Read the model definition and answer for the solid it produces. Units are mm, in the model's axes. Coordinates: 2 decimals unless noted, no trailing zeros. Loops run counter-clockwise (first coordinate to the right, second up) from the corner with the lowest first, then second, coordinate; pieces in that order, holes last. Notation, with made-up numbers: M -36.75,-23 L -0.75,-23 A16 ccw -0.75,-11 Z; hole C -13,24 d10. An arc over 180 degrees is marked long. One line per item, written item: value. Start each with the question number.
1. Flat-ended cylindrical pins translate along their axes: pin 1 (3 mm diameter, centred on x = 7, z = 5.5, fed in from -Y); pin 2 (12 mm diameter, centred on x = -2.5, y = -2.5, fed in from +Z); pin 3 (1.5 mm diameter, centred on y = -8, z = 1.5, fed in from -X). Find the tip coordinate at first contact, or state that the pin passes through.
2. The part is cut by section D-D (y = -3). State how many separate pieces and enclosed holes the cut face has, then the cut area to 3 significant figures.
3. Determine the mould class of faces 1 (the face through (-7, -11, 10)), 2 (the face through (-2.764, -12.447, 4.93)) for opening direction Y: +Y half, -Y half, draft (parallel to the pull), parting line (faces both ways), or undercut.
4. The part is cut by section A-A (x = 0). Write down the section's boundary in (y, z).
5. The part is cut by section C-C (x = 8.25). Write down the section's boundary in (y, z).
6. Consider probe 1 along Y at (x, z) = (0, 2.5); probe 2 along X at (y, z) = (4.5, 8); probe 3 along Z at (x, y) = (8, 7.75). Determine where each line is inside the solid, lowest interval first.
```python
from build123d import *

# Parameters (mm, degrees)
SKETCH1_R           = 15
SKETCH1_R_2         = 12.75
BOSS_EXTRUDE1_DEPTH = 10
SKETCH2_R           = 15
BOSS_EXTRUDE2_DEPTH = 0.25
FILLET1_R           = 3


with BuildPart() as part:
    # Sketch1 → Boss-Extrude1 (new body)
    with BuildSketch(Plane.XY):
        Circle(SKETCH1_R)
        Circle(SKETCH1_R_2, mode=Mode.SUBTRACT)
    extrude(amount=BOSS_EXTRUDE1_DEPTH)

    # Sketch2 → Boss-Extrude2 (add)
    with BuildSketch(Plane.XY):
        Circle(SKETCH2_R)
        with BuildLine():
            Line((5.922042758, 5.03811235), (5.03811235, 5.922042758))
            Line((5.03811235, 5.922042758), (1.502578444, 9.457576664))
            ThreePointArc((1.502578444, 9.457576664), (1.149025054, 9.457576664), (1.149025054, 9.104023274))
            Line((1.149025054, 9.104023274), (4.684558959, 5.568489368))
            Line((4.684558959, 5.568489368), (5.568489368, 4.684558959))
            Line((5.568489368, 4.684558959), (9.104023274, 1.149025054))
            ThreePointArc((9.104023274, 1.149025054), (9.457576664, 1.149025054), (9.457576664, 1.502578444))
            Line((9.457576664, 1.502578444), (5.922042758, 5.03811235))
        make_face(mode=Mode.SUBTRACT)
        with BuildLine():
            Line((6.346306827, 5.462376419), (9.881840733, 1.926842513))
            ThreePointArc((9.881840733, 1.926842513), (9.881840733, 0.724760985), (8.679759205, 0.724760985))
            Line((8.679759205, 0.724760985), (5.144225299, 4.260294891))
            Line((5.144225299, 4.260294891), (4.684605891, 3.800675483))
            ThreePointArc((4.684605891, 3.800675483), (6.032467694, 0), (4.684605891, -3.800675483))
            Line((4.684605891, -3.800675483), (5.144225299, -4.260294891))
            Line((5.144225299, -4.260294891), (8.679759205, -0.724760985))
            ThreePointArc((8.679759205, -0.724760985), (9.881840733, -0.724760985), (9.881840733, -1.926842513))
            Line((9.881840733, -1.926842513), (6.346306827, -5.462376419))
            Line((6.346306827, -5.462376419), (6.805926235, -5.921995827))
            Line((6.805926235, -5.921995827), (12.727922061, 0))
            Line((12.727922061, 0), (6.805926235, 5.921995827))
            Line((6.805926235, 5.921995827), (6.346306827, 5.462376419))
        make_face(mode=Mode.SUBTRACT)
        with BuildLine():
            Line((5.462376419, 6.346306827), (1.926842513, 9.881840733))
            ThreePointArc((1.926842513, 9.881840733), (0.724760985, 9.881840733), (0.724760985, 8.679759205))
            Line((0.724760985, 8.679759205), (4.260294891, 5.144225299))
            Line((4.260294891, 5.144225299), (3.800675483, 4.684605891))
            ThreePointArc((3.800675483, 4.684605891), (0, 6.032467694), (-3.800675483, 4.684605891))
            Line((-3.800675483, 4.684605891), (-4.260294891, 5.144225299))
            Line((-4.260294891, 5.144225299), (-0.724760985, 8.679759205))
            ThreePointArc((-0.724760985, 8.679759205), (-0.724760985, 9.881840733), (-1.926842513, 9.881840733))
            Line((-1.926842513, 9.881840733), (-5.462376419, 6.346306827))
            Line((-5.462376419, 6.346306827), (-5.921995827, 6.805926235))
            Line((-5.921995827, 6.805926235), (0, 12.727922061))
            Line((0, 12.727922061), (5.921995827, 6.805926235))
            Line((5.921995827, 6.805926235), (5.462376419, 6.346306827))
        make_face(mode=Mode.SUBTRACT)
        with BuildLine():
            Line((-5.568489368, 4.684558959), (-9.104023274, 1.149025054))
            ThreePointArc((-9.104023274, 1.149025054), (-9.457576664, 1.149025054), (-9.457576664, 1.502578444))
            Line((-9.457576664, 1.502578444), (-5.922042758, 5.03811235))
            Line((-5.922042758, 5.03811235), (-5.03811235, 5.922042758))
            Line((-5.03811235, 5.922042758), (-1.502578444, 9.457576664))
            ThreePointArc((-1.502578444, 9.457576664), (-1.149025054, 9.457576664), (-1.149025054, 9.104023274))
            Line((-1.149025054, 9.104023274), (-4.684558959, 5.568489368))
            Line((-4.684558959, 5.568489368), (-5.568489368, 4.684558959))
        make_face(mode=Mode.SUBTRACT)
        with BuildLine():
            Line((-6.346306827, 5.462376419), (-6.805926235, 5.921995827))
            Line((-6.805926235, 5.921995827), (-12.727922061, 0))
            Line((-12.727922061, 0), (-6.805926235, -5.921995827))
            Line((-6.805926235, -5.921995827), (-6.346306827, -5.462376419))
            Line((-6.346306827, -5.462376419), (-9.881840733, -1.926842513))
            ThreePointArc((-9.881840733, -1.926842513), (-9.881840733, -0.724760985), (-8.679759205, -0.724760985))
            Line((-8.679759205, -0.724760985), (-5.144225299, -4.260294891))
            Line((-5.144225299, -4.260294891), (-4.684605891, -3.800675483))
            ThreePointArc((-4.684605891, -3.800675483), (-6.032467694, 0), (-4.684605891, 3.800675483))
            Line((-4.684605891, 3.800675483), (-5.144225299, 4.260294891))
            Line((-5.144225299, 4.260294891), (-8.679759205, 0.724760985))
            ThreePointArc((-8.679759205, 0.724760985), (-9.881840733, 0.724760985), (-9.881840733, 1.926842513))
            Line((-9.881840733, 1.926842513), (-6.346306827, 5.462376419))
        make_face(mode=Mode.SUBTRACT)
        with BuildLine():
            Line((5.462376419, -6.346306827), (5.921995827, -6.805926235))
            Line((5.921995827, -6.805926235), (0, -12.727922061))
            Line((0, -12.727922061), (-5.921995827, -6.805926235))
            Line((-5.921995827, -6.805926235), (-5.462376419, -6.346306827))
            Line((-5.462376419, -6.346306827), (-1.926842513, -9.881840733))
            ThreePointArc((-1.926842513, -9.881840733), (-0.724760985, -9.881840733), (-0.724760985, -8.679759205))
            Line((-0.724760985, -8.679759205), (-4.260294891, -5.144225299))
            Line((-4.260294891, -5.144225299), (-3.800675483, -4.684605891))
            ThreePointArc((-3.800675483, -4.684605891), (0, -6.032467694), (3.800675483, -4.684605891))
            Line((3.800675483, -4.684605891), (4.260294891, -5.144225299))
            Line((4.260294891, -5.144225299), (0.724760985, -8.679759205))
            ThreePointArc((0.724760985, -8.679759205), (0.724760985, -9.881840733), (1.926842513, -9.881840733))
            Line((1.926842513, -9.881840733), (5.462376419, -6.346306827))
        make_face(mode=Mode.SUBTRACT)
        with BuildLine():
            Line((5.568489368, -4.684558959), (9.104023274, -1.149025054))
            ThreePointArc((9.104023274, -1.149025054), (9.457576664, -1.149025054), (9.457576664, -1.502578444))
            Line((9.457576664, -1.502578444), (5.922042758, -5.03811235))
            Line((5.922042758, -5.03811235), (5.03811235, -5.922042758))
            Line((5.03811235, -5.922042758), (1.502578444, -9.457576664))
            ThreePointArc((1.502578444, -9.457576664), (1.149025054, -9.457576664), (1.149025054, -9.104023274))
            Line((1.149025054, -9.104023274), (4.684558959, -5.568489368))
            Line((4.684558959, -5.568489368), (5.568489368, -4.684558959))
        make_face(mode=Mode.SUBTRACT)
        with BuildLine():
            Line((-5.568489368, -4.684558959), (-4.684558959, -5.568489368))
            Line((-4.684558959, -5.568489368), (-1.149025054, -9.104023274))
            ThreePointArc((-1.149025054, -9.104023274), (-1.149025054, -9.457576664), (-1.502578444, -9.457576664))
            Line((-1.502578444, -9.457576664), (-5.03811235, -5.922042758))
            Line((-5.03811235, -5.922042758), (-5.922042758, -5.03811235))
            Line((-5.922042758, -5.03811235), (-9.457576664, -1.502578444))
            ThreePointArc((-9.457576664, -1.502578444), (-9.457576664, -1.149025054), (-9.104023274, -1.149025054))
            Line((-9.104023274, -1.149025054), (-5.568489368, -4.684558959))
        make_face(mode=Mode.SUBTRACT)
    extrude(amount=-BOSS_EXTRUDE2_DEPTH)

    # Fillet1
    fillet1_edges = [part.edges().sort_by_distance(p)[0] for p in [
        (0, -12.727922061, -0.125),
        (-12.727922061, 0, -0.125),
        (0, 12.727922061, -0.125),
        (12.727922061, 0, -0.125),
    ]]
    fillet(fillet1_edges, radius=FILLET1_R)


solid = part.part
```
Answer block:
1. pin 1: stops at y = -13.96
1. pin 2: stops at z = 0
1. pin 3: stops at x = -13.13
2. separate pieces: 7
2. enclosed holes: 0
2. area: 52.0 mm2
3. face 1: draft
3. face 2: undercut
4. outline: M -15,-0.25 L -11.49,-0.25 L -11.49,0 L -12.75,0 L -12.75,10 L -15,10 Z; M -6.03,-0.25 L 6.03,-0.25 L 6.03,0 L -6.03,0 Z; M 11.49,-0.25 L 15,-0.25 L 15,10 L 12.75,10 L 12.75,0 L 11.49,0 Z
5. outline: M -12.53,-0.25 L -4.48,-0.25 L -4.48,0 L -9.72,0 L -9.72,10 L -12.53,10 Z; M -3.56,-0.25 L -2.71,-0.25 L -2.71,0 L -3.56,0 Z; M -2,-0.25 L -1.15,-0.25 L -1.15,0 L -2,0 Z; M 1.15,-0.25 L 2,-0.25 L 2,0 L 1.15,0 Z; M 2.71,-0.25 L 3.56,-0.25 L 3.56,0 L 2.71,0 Z; M 4.48,-0.25 L 12.53,-0.25 L 12.53,10 L 9.72,10 L 9.72,0 L 4.48,0 Z
6. probe 1: y = -15 to -12.75, 12.75 to 15
6. probe 2: x = -14.31 to -11.93, 11.93 to 14.31
6. probe 3: z = -0.25 to 0
